Input: part model. Units: mm. Frame: model coordinates. A direction names the side the tool comes from. Round coordinates to 2 decimals unless told otherwise and drop trailing zeros. Write each loop counter-clockwise with the first axis right and the second up, starting at its lowest first coordinate (ties: lowest second). Pieces come first, ordered by that corner, then holes. Notation, with made-up numbers: (15, 43.5) -> (20, 43.5) arc R26 cw to (20, 68.5) -> close; hole circle Ø5 at (53, 66). An arc over 180 degrees is marked (long way). Write item = value, one per line.
```python
from build123d import *

# Parameters (mm, degrees)
SKIZZE1_R                       = 2.15
AUFSATZ_LINEAR_AUSTRAGEN1_DEPTH = 102.5


with BuildPart() as part:
    # Skizze1 → Aufsatz-Linear austragen1 (new body)
    with BuildSketch(Plane.XY.offset(100)):
        with BuildLine():
            Line((12.499999989, 1.499999999), (12.499999989, 0.800000002))
            ThreePointArc((12.499999989, 0.800000002), (12.734314564, 0.234314576), (13.299999991, 0))
            Line((13.299999991, 0), (18, 0))
            ThreePointArc((18, 0), (19.414213562, 0.585786438), (20, 2))
            Line((20, 2), (20, 6.700000003))
            ThreePointArc((20, 6.700000003), (19.765685425, 7.265685427), (19.2, 7.500000003))
            Line((19.2, 7.500000003), (18.499999995, 7.500000003))
            ThreePointArc((18.499999995, 7.500000003), (18.287867961, 7.412132037), (18.199999995, 7.200000003))
            Line((18.199999995, 7.200000003), (18.199999995, 5.082411607))
            ThreePointArc((18.199999995, 5.082411607), (17.686138517, 4.313363558), (16.778984491, 4.493807713))
            Line((16.778984491, 4.493807713), (14.528679651, 6.744112553))
            ThreePointArc((14.528679651, 6.744112553), (13.878361397, 7.717382599), (13.649999995, 8.865432896))
            Line((13.649999995, 8.865432896), (13.649999995, 11.134567106))
            ThreePointArc((13.649999995, 11.134567106), (13.878361397, 12.282617403), (14.528679651, 13.255887449))
            Line((14.528679651, 13.255887449), (16.778984493, 15.506192291))
            ThreePointArc((16.778984493, 15.506192291), (17.686138518, 15.686636446), (18.199999995, 14.917588398))
            Line((18.199999995, 14.917588398), (18.199999995, 12.800000001))
            ThreePointArc((18.199999995, 12.800000001), (18.287867961, 12.587867966), (18.499999996, 12.5))
            Line((18.499999996, 12.5), (19.199999998, 12.5))
            ThreePointArc((19.199999998, 12.5), (19.765685424, 12.734314576), (20, 13.300000003))
            Line((20, 13.300000003), (20, 18))
            ThreePointArc((20, 18), (19.414213562, 19.414213562), (18, 20))
            Line((18, 20), (13.299999989, 20))
            ThreePointArc((13.299999989, 20), (12.734314564, 19.765685425), (12.499999989, 19.2))
            Line((12.499999989, 19.2), (12.499999989, 18.499999999))
            ThreePointArc((12.499999989, 18.499999999), (12.587867954, 18.287867964), (12.799999989, 18.199999999))
            Line((12.799999989, 18.199999999), (14.917588395, 18.199999999))
            ThreePointArc((14.917588395, 18.199999999), (15.686636445, 17.68613852), (15.50619229, 16.778984493))
            Line((15.50619229, 16.778984493), (13.255887454, 14.528679658))
            ThreePointArc((13.255887454, 14.528679658), (12.282617408, 13.878361404), (11.134567111, 13.650000002))
            Line((11.134567111, 13.650000002), (8.865432888, 13.650000002))
            ThreePointArc((8.865432888, 13.650000002), (7.717382592, 13.878361404), (6.744112546, 14.528679658))
            Line((6.744112546, 14.528679658), (4.493807706, 16.778984498))
            ThreePointArc((4.493807706, 16.778984498), (4.313363551, 17.686138522), (5.082411599, 18.199999999))
            Line((5.082411599, 18.199999999), (7.199999999, 18.199999999))
            ThreePointArc((7.199999999, 18.199999999), (7.412132034, 18.287867965), (7.5, 18.5))
            Line((7.5, 18.5), (7.5, 19.199999998))
            ThreePointArc((7.5, 19.199999998), (7.265685424, 19.765685424), (6.699999997, 20))
            Line((6.699999997, 20), (2, 20))
            ThreePointArc((2, 20), (0.585786438, 19.414213562), (0, 18))
            Line((0, 18), (0, 13.3))
            ThreePointArc((0, 13.3), (0.234314575, 12.734314575), (0.8, 12.5))
            Line((0.8, 12.5), (1.500000004, 12.5))
            ThreePointArc((1.500000004, 12.5), (1.712132038, 12.587867966), (1.800000004, 12.8))
            Line((1.800000004, 12.8), (1.800000004, 14.917588391))
            ThreePointArc((1.800000004, 14.917588391), (2.313861482, 15.68663644), (3.221015508, 15.506192285))
            Line((3.221015508, 15.506192285), (5.471320345, 13.255887449))
            ThreePointArc((5.471320345, 13.255887449), (6.121638599, 12.282617402), (6.350000001, 11.134567106))
            Line((6.350000001, 11.134567106), (6.350000001, 8.865432891))
            ThreePointArc((6.350000001, 8.865432891), (6.121638599, 7.717382594), (5.471320345, 6.744112548))
            Line((5.471320345, 6.744112548), (3.221015505, 4.493807708))
            ThreePointArc((3.221015505, 4.493807708), (2.313861481, 4.313363554), (1.800000004, 5.082411601))
            Line((1.800000004, 5.082411601), (1.800000004, 7.200000001))
            ThreePointArc((1.800000004, 7.200000001), (1.712132038, 7.412132036), (1.500000003, 7.500000002))
            Line((1.500000003, 7.500000002), (0.800000003, 7.500000002))
            ThreePointArc((0.800000003, 7.500000002), (0.234314576, 7.265685427), (0, 6.7))
            Line((0, 6.7), (0, 2))
            ThreePointArc((0, 2), (0.585786438, 0.585786438), (2, 0))
            Line((2, 0), (6.7, 0))
            ThreePointArc((6.7, 0), (7.265685425, 0.234314575), (7.5, 0.8))
            Line((7.5, 0.8), (7.5, 1.5))
            ThreePointArc((7.5, 1.5), (7.412132034, 1.712132034), (7.2, 1.8))
            Line((7.2, 1.8), (5.0824116, 1.8))
            ThreePointArc((5.0824116, 1.8), (4.313363551, 2.313861478), (4.493807706, 3.221015504))
            Line((4.493807706, 3.221015504), (6.744112546, 5.471320344))
            ThreePointArc((6.744112546, 5.471320344), (7.717382592, 6.121638598), (8.865432889, 6.35))
            Line((8.865432889, 6.35), (11.134567106, 6.35))
            ThreePointArc((11.134567106, 6.35), (12.282617403, 6.121638598), (13.255887449, 5.471320344))
            Line((13.255887449, 5.471320344), (15.506192291, 3.221015502))
            ThreePointArc((15.506192291, 3.221015502), (15.686636446, 2.313861477), (14.917588398, 1.8))
            Line((14.917588398, 1.8), (12.79999999, 1.8))
            ThreePointArc((12.79999999, 1.8), (12.587867955, 1.712132034), (12.499999989, 1.499999999))
        make_face()
        with Locations((10, 10)):
            Circle(SKIZZE1_R, mode=Mode.SUBTRACT)
    extrude(amount=-AUFSATZ_LINEAR_AUSTRAGEN1_DEPTH)


solid = part.part
```
1) Cut plane A-A (y = 10). Return the cut outline in (x, z), and give its area (4 significant figures).
Solutions:
outline = (6.35, -2.5) -> (7.85, -2.5) -> (7.85, 100) -> (6.35, 100) -> close; (12.15, -2.5) -> (13.65, -2.5) -> (13.65, 100) -> (12.15, 100) -> close
area = 307.5 mm^2
2) Line query: L1, parallel to Y at x = 6.75, z = 14; L2, parallel to Y at x = 10, z = 77; L3, parallel to X at y = 13.5, z = 87.5. Output: solid intervals per line, ascending. Write a range as from..to.
Solutions:
L1 = 0..1.8, 5.48..14.52, 18.2..20
L2 = 6.35..7.85, 12.15..13.65
L3 = 0..1.8, 5.23..14.77, 18.2..20
3) Draft query along Y for faces 4 (the face through (0.6, 19.43, 49.47)), 5 (the face through (19.4, 0.57, 49.47)), 6 (the face through (0, 4, 49)), 7 (the face through (6.35, 10, 49)). Return one class per face: +Y half, -Y half, draft (parallel to the pull), parting line (faces both ways), or undercut.
Solutions:
face_4 = +Y half
face_5 = -Y half
face_6 = draft
face_7 = undercut
4) First-contact query: P1, Ø0.8, axis at y = 1, z = 62.5, coming from the +X side; P2, Ø0.6, axis at y = 19, z = 27, coming from the -X side; P3, Ø2.5, axis at y = 9.5, z = 73, coming from the +X side. Flat tips, straight axial feed; report the tip coordinate or a pass-through.
Solutions:
P1 = 19.91
P2 = 0.13
P3 = 13.71
5) Access query for faces 1 (the face through (15.64, 14.37, 49.47)), 2 (the face through (19.43, 19.4, 49.47)), 3 (the face through (13.65, 10, 49)). Directions: +Z, -Z, +X, -X, +Y, -Y. A direction counts if a zero-diameter tool reaches every point of the face in a straight line with its end or side. Return the directions, or none.
Solutions:
face_1 = +Z, -Z
face_2 = +Z, -Z, +X, +Y
face_3 = +Z, -Z, +X
